Read the model definition and answer for the solid it produces. Units are mm, in the model's axes. A direction names the side the tool comes from. Coordinates: 2 decimals unless noted, no trailing zeros. Loops run counter-clockwise (first coordinate to the right, second up) from the corner with the lowest first, then second, coordinate; pieces in that order, holes last. Notation, with made-up numbers: (32, 64) -> (71, 64) arc R21 ccw to (71, 73) -> close; hole circle Ø11 at (68.25, 17). An arc over 180 degrees is marked (long way). Answer as a JSON object with one key per item and string values. Group by question number.
1) Flat-ended cylindrical pins translate along their axes: P1, Ø1.5, axis at x = 0, z = 0, coming from the -Y side; P2, Ø1, axis at x = 8.5, z = -1.5, coming from the +Y side; P3, Ø0.8, axis at x = 9.5, y = 5, coming from the +Z side; P4, Ø1, axis at x = 1, y = 7.5, coming from the -Z side. Find the tip coordinate at first contact, or state that the pin passes through.
2) Section C-C, the plane x = 5.5 is taken. Give the vertices of the cut face in (y, z).
3) Which of the six approach directions +Z, -Z, +X, -X, +Y, -Y give full straight-line access (tool end or side, diameter ignored) to faces 1 (the face through (9, 5, 1)), 2 (the face through (-3.497, 6.877, -0.154)), 3 (the face through (1, 5.75, 1))?
4) Determine the mould class of faces 4 (the face through (-2, 8.5, 2)), 5 (the face through (5.63, 5.26, -2.16)), 6 (the face through (-0.29, 4.99, -2.23)) for opening direction Z: released by +Z, released by -Z, zero draft, split by the parting line, or undercut.
5) Consider probe 1 along Z at (x, y) = (0, 4.6); probe 2 along X at (y, z) = (4.7, 0); probe 3 along X at (y, z) = (6.15, 0). Determine where each line is inside the solid, lowest interval first. Write a range as [from, to].
6) Section B-B, the plane z = -3 is taken. Give the vertices of the cut face in (x, y).
7) Section A-A, the plane y = 4.65 is taken. Give the vertices of the cut face in (x, z) (3 decimals), plus the area to 3 significant figures.
from build123d import *

# Parameters (mm, degrees)
SKETCH1_R           = 3.5
SKETCH1_R_2         = 2.5
BOSS_EXTRUDE1_DEPTH = 2.25
BOSS_EXTRUDE4_DEPTH = 2.25
BOSS_EXTRUDE2_START = 2.25
BOSS_EXTRUDE2_DEPTH = 2
SKETCH3_R           = 3.5
SKETCH3_R_2         = 1.25
BOSS_EXTRUDE3_DEPTH = 2
SKETCH4_R           = 2.25
CUT_EXTRUDE1_DEPTH  = 1.5


with BuildPart() as part:
    # Sketch1 → Boss-Extrude1 (new body)
    with BuildSketch(Plane(origin=(0, 0, 0), x_dir=(1, 0, 0), z_dir=(0, 1, 0))):
        Circle(SKETCH1_R)
        Circle(SKETCH1_R_2, mode=Mode.SUBTRACT)
    extrude(amount=BOSS_EXTRUDE1_DEPTH)

    # Sketch6 → Boss-Extrude4 (add)
    with BuildSketch(Plane.XZ):
        with BuildLine():
            Line((0.434120444, 2.462019383), (0.408073218, 2.31429822))
            ThreePointArc((0.408073218, 2.31429822), (0.551444891, 2.284383622), (0.69267466, 2.245596094))
            Line((0.69267466, 2.245596094), (0.736887936, 2.388932014))
            ThreePointArc((0.736887936, 2.388932014), (0.586643501, 2.430195342), (0.434120444, 2.462019383))
        make_face()
        with BuildLine():
            Line((1.140526643, 2.224679522), (1.072095045, 2.091198751))
            ThreePointArc((1.072095045, 2.091198751), (1.200279635, 2.020353632), (1.323802136, 1.94166112))
            Line((1.323802136, 1.94166112), (1.408300145, 2.065596936))
            ThreePointArc((1.408300145, 2.065596936), (1.276893228, 2.149312375), (1.140526643, 2.224679522))
        make_face()
        with BuildLine():
            Line((1.745592045, 1.789667123), (1.640856523, 1.682287096))
            ThreePointArc((1.640856523, 1.682287096), (1.742464265, 1.576806356), (1.837303984, 1.465201034))
            Line((1.837303984, 1.465201034), (1.954578706, 1.558724505))
            ThreePointArc((1.954578706, 1.558724505), (1.853685389, 1.67745357), (1.745592045, 1.789667123))
        make_face()
        with BuildLine():
            Line((2.195553933, 1.195634947), (2.063820697, 1.12389685))
            ThreePointArc((2.063820697, 1.12389685), (2.1298233, 0.993152915), (2.187553309, 0.858551407))
            Line((2.187553309, 0.858551407), (2.327184372, 0.913352561))
            ThreePointArc((2.327184372, 0.913352561), (2.265769468, 1.056545654), (2.195553933, 1.195634947))
        make_face()
        with BuildLine():
            Line((2.45043122, 0.495365358), (2.303405346, 0.465643437))
            ThreePointArc((2.303405346, 0.465643437), (2.327938187, 0.32125348), (2.343428923, 0.17561572))
            Line((2.343428923, 0.17561572), (2.493009493, 0.186825234))
            ThreePointArc((2.493009493, 0.186825234), (2.476529986, 0.341759021), (2.45043122, 0.495365358))
        make_face()
        with BuildLine():
            Line((2.487576938, -0.248919616), (2.338322322, -0.23398444))
            ThreePointArc((2.338322322, -0.23398444), (2.31920555, -0.379190737), (2.291080594, -0.522924195))
            Line((2.291080594, -0.522924195), (2.43731978, -0.556302335))
            ThreePointArc((2.43731978, -0.556302335), (2.467239947, -0.403394402), (2.487576938, -0.248919616))
        make_face()
        with BuildLine():
            Line((2.30369053, -0.971086991), (2.165469098, -0.912821771))
            ThreePointArc((2.165469098, -0.912821771), (2.104401323, -1.045942193), (2.035159699, -1.175))
            Line((2.035159699, -1.175), (2.165063509, -1.25))
            ThreePointArc((2.165063509, -1.25), (2.238724812, -1.112704461), (2.30369053, -0.971086991))
        make_face()
        with BuildLine():
            Line((1.915111108, -1.606969024), (1.800204441, -1.510550883))
            ThreePointArc((1.800204441, -1.510550883), (1.702611803, -1.619757095), (1.598405934, -1.722671899))
            Line((1.598405934, -1.722671899), (1.700431844, -1.83262968))
            ThreePointArc((1.700431844, -1.83262968), (1.811289152, -1.723145846), (1.915111108, -1.606969024))
        make_face()
        with BuildLine():
            Line((1.35636566, -2.100064808), (1.27498372, -1.974060919))
            ThreePointArc((1.27498372, -1.974060919), (1.149537753, -2.049649471), (1.019626787, -2.11727684))
            Line((1.019626787, -2.11727684), (1.084709348, -2.25242217))
            ThreePointArc((1.084709348, -2.25242217), (1.222912503, -2.180478161), (1.35636566, -2.100064808))
        make_face()
        with BuildLine():
            Line((0.67710117, -2.406560617), (0.6364751, -2.26216698))
            ThreePointArc((0.6364751, -2.26216698), (0.494322228, -2.297421497), (0.350249326, -2.323752442))
            Line((0.350249326, -2.323752442), (0.372605665, -2.472077066))
            ThreePointArc((0.372605665, -2.472077066), (0.525874711, -2.444065422), (0.67710117, -2.406560617))
        make_face()
        with BuildLine():
            Line((-0.062326729, -2.499222955), (-0.058587126, -2.349269578))
            ThreePointArc((-0.058587126, -2.349269578), (-0.204815995, -2.341057541), (-0.350249326, -2.323752442))
            Line((-0.350249326, -2.323752442), (-0.372605665, -2.472077066))
            ThreePointArc((-0.372605665, -2.472077066), (-0.217889357, -2.490486745), (-0.062326729, -2.499222955))
        make_face()
        with BuildLine():
            Line((-0.796216626, -2.369818365), (-0.748443628, -2.227629263))
            ThreePointArc((-0.748443628, -2.227629263), (-0.885755419, -2.176680348), (-1.019626787, -2.11727684))
            Line((-1.019626787, -2.11727684), (-1.084709348, -2.25242217))
            ThreePointArc((-1.084709348, -2.25242217), (-0.942292999, -2.315617392), (-0.796216626, -2.369818365))
        make_face()
        with BuildLine():
            Line((-1.459359181, -2.029845014), (-1.37179763, -1.908054313))
            ThreePointArc((-1.37179763, -1.908054313), (-1.487991587, -1.818895554), (-1.598405934, -1.722671899))
            Line((-1.598405934, -1.722671899), (-1.700431844, -1.83262968))
            ThreePointArc((-1.700431844, -1.83262968), (-1.582969773, -1.934995271), (-1.459359181, -2.029845014))
        make_face()
        with BuildLine():
            Line((-1.992831268, -1.509511026), (-1.873261392, -1.418940364))
            ThreePointArc((-1.873261392, -1.418940364), (-1.958013172, -1.299493909), (-2.035159699, -1.175))
            Line((-2.035159699, -1.175), (-2.165063509, -1.25))
            ThreePointArc((-2.165063509, -1.25), (-2.082992736, -1.382440328), (-1.992831268, -1.509511026))
        make_face()
        with BuildLine():
            Line((-2.349231552, -0.855050358), (-2.208277659, -0.803747337))
            ThreePointArc((-2.208277659, -0.803747337), (-2.254056694, -0.664626526), (-2.291080594, -0.522924195))
            Line((-2.291080594, -0.522924195), (-2.43731978, -0.556302335))
            ThreePointArc((-2.43731978, -0.556302335), (-2.397932653, -0.707049496), (-2.349231552, -0.855050358))
        make_face()
        with BuildLine():
            Line((-2.496892303, -0.124614714), (-2.347078765, -0.117137831))
            ThreePointArc((-2.347078765, -0.117137831), (-2.349817387, 0.029295839), (-2.343428923, 0.17561572))
            Line((-2.343428923, 0.17561572), (-2.493009493, 0.186825234))
            ThreePointArc((-2.493009493, 0.186825234), (-2.499805731, 0.031165786), (-2.496892303, -0.124614714))
        make_face()
        with BuildLine():
            Line((-2.422693216, 0.616893494), (-2.277331623, 0.579879885))
            ThreePointArc((-2.277331623, 0.579879885), (-2.236786494, 0.720615141), (-2.187553309, 0.858551407))
            Line((-2.187553309, 0.858551407), (-2.327184372, 0.913352561))
            ThreePointArc((-2.327184372, 0.913352561), (-2.3795601, 0.766611852), (-2.422693216, 0.616893494))
        make_face()
        with BuildLine():
            Line((-2.133227204, 1.303588008), (-2.005233572, 1.225372728))
            ThreePointArc((-2.005233572, 1.225372728), (-1.925007304, 1.347904625), (-1.837303984, 1.465201034))
            Line((-1.837303984, 1.465201034), (-1.954578706, 1.558724505))
            ThreePointArc((-1.954578706, 1.558724505), (-2.047880111, 1.433941091), (-2.133227204, 1.303588008))
        make_face()
        with BuildLine():
            Line((-1.654214594, 1.874453007), (-1.554961718, 1.761985827))
            ThreePointArc((-1.554961718, 1.761985827), (-1.442182768, 1.855426869), (-1.323802136, 1.94166112))
            Line((-1.323802136, 1.94166112), (-1.408300145, 2.065596936))
            ThreePointArc((-1.408300145, 2.065596936), (-1.534236987, 1.973858371), (-1.654214594, 1.874453007))
        make_face()
        with BuildLine():
            Line((-1.028217758, 2.278764631), (-0.966524692, 2.142038753))
            ThreePointArc((-0.966524692, 2.142038753), (-0.831213964, 2.198086292), (-0.69267466, 2.245596094))
            Line((-0.69267466, 2.245596094), (-0.736887936, 2.388932014))
            ThreePointArc((-0.736887936, 2.388932014), (-0.884270174, 2.338389672), (-1.028217758, 2.278764631))
        make_face()
        with BuildLine():
            Line((-0.310859262, 2.480598017), (-0.292207706, 2.331762136))
            ThreePointArc((-0.292207706, 2.331762136), (-0.146388151, 2.345436102), (0, 2.35))
            Line((0, 2.35), (0, 2.5))
            ThreePointArc((0, 2.5), (-0.155732076, 2.49514479), (-0.310859262, 2.480598017))
        make_face()
    extrude(amount=-BOSS_EXTRUDE4_DEPTH)



with BuildPart() as body_2:
    # Sketch2 → Boss-Extrude2 (new body)
    with BuildSketch(Plane(origin=(0, 0, 0), x_dir=(1, 0, 0), z_dir=(0, 1, 0)).offset(BOSS_EXTRUDE2_START)):
        with BuildLine():
            Line((10.25, 0.968245837), (0.875, 3.388860428))
            ThreePointArc((0.875, 3.388860428), (3.497755962, 0.12531253), (1.115267765, -3.317556))
            Line((1.115267765, -3.317556), (7.544056202, -1.156380571))
            ThreePointArc((7.544056202, -1.156380571), (8.015674844, -1.039353256), (8.5, -1))
            Line((8.5, -1), (10, -1))
            ThreePointArc((10, -1), (10.992029696, -0.126004292), (10.25, 0.968245837))
        make_face()
    extrude(amount=BOSS_EXTRUDE2_DEPTH)


with BuildPart() as part_1:
    add(part.part)

    add(body_2.part)  # Boss-Extrude3 merges body 2
    # Sketch3 → Boss-Extrude3 (add)
    with BuildSketch(Plane(origin=(0, 2.25, 0), x_dir=(1, 0, 0), z_dir=(0, 1, 0))):
        Circle(SKETCH3_R)
        Circle(SKETCH3_R_2, mode=Mode.SUBTRACT)
    extrude(amount=BOSS_EXTRUDE3_DEPTH)

    # Sketch4 → Cut-Extrude1 (cut)
    with BuildSketch(Plane(origin=(0, 4.25, 0), x_dir=(1, 0, 0), z_dir=(0, 1, 0))):
        Circle(SKETCH4_R)
    extrude(amount=-CUT_EXTRUDE1_DEPTH, mode=Mode.SUBTRACT)


with BuildPart() as body_2_2:
    # Mirror1: mirrored copy
    add(part_1.part.mirror(Plane(origin=(3.303845643, 4.25, -0.0910361), x_dir=(0, 0, 1), z_dir=(0, 1, 0))))


solid = body_2_2.part
Determined:
{
 "1": {"P1": "through", "P2": "y = 6.25", "P3": "z = 1", "P4": "z = -3.46"},
 "2": {"outline": "(4.25, -2.19) -> (6.25, -2.19) -> (6.25, 1.84) -> (4.25, 1.84) -> close"},
 "3": {"face 1": "+Z, +X, +Y, -Y", "face 2": "+Y", "face 3": "-Y"},
 "4": {"face 4": "zero draft", "face 5": "released by -Z", "face 6": "undercut"},
 "5": {"probe 1": "[-3.5, -2.25], [2.25, 3.5]", "probe 2": "[-3.5, -2.25], [2.25, 11]", "probe 3": "[-3.5, -1.25], [1.25, 11]"},
 "6": {"outline": "(-1.8, 4.25) -> (2.38, 4.25) -> (2.38, 6.25) -> (1.8, 6.25) -> (1.8, 8.5) -> (-1.8, 8.5) -> close"},
 "7": {"outline": "(0.875, -3.389) -> (10.25, -0.968) arc R1 ccw to (10, 1) -> (8.5, 1) arc R3 cw to (7.544, 1.156) -> (1.115, 3.318) arc R3.5 ccw (long way) to start; hole circle Ø4.5 at (0, 0)", "area": "48.8 mm²"}
}
